Read the model definition and answer for the solid it produces. Units are mm, in the model's axes. A direction names the side the tool comes from. Coordinates: 2 decimals unless noted, no trailing zeros. Write each loop counter-clockwise with the first axis right and the second up, starting at its lowest first coordinate (ties: lowest second). Pieces come first, ordered by that corner, then holes. Notation, with made-up numbers: (-28.5, 50.5) -> (27.5, 50.5) arc R29 ccw to (27.5, 81.5) -> close; hole circle Ø11 at (-25, -36.75). An arc over 180 degrees is marked (long way). Use CSV: the item, a comma, the result in double quotes. Start each with the question number.
from build123d import *

# Parameters (mm, degrees)
BOSS_EXTRUDE1_DEPTH        = 2.5
SKETCH6_W                  = 0.64
SKETCH6_H                  = 0.64
CUT_EXTRUDE1_DEPTH         = 2.5
SKETCH15_W                 = 0.64
SKETCH15_H                 = 0.64
CHAMFER4_SIZE              = 0.12
LPATTERN5_COUNT            = 2
LPATTERN5_PITCH            = 2.5
CHAMFER4_OF_LPATTERN5_SIZE = 0.12


with BuildPart() as part:
    # Sketch4 → Boss-Extrude1 (new body)
    with BuildSketch(Plane(origin=(0, 0, 0), x_dir=(1, 0, 0), z_dir=(0, 1, 0))):
        Polygon((-2.37, -0.9), (-2.37, -0.95), (-2.07, -1.25), (-0.47, -1.25), (-0.17, -0.95), (-0.17, -0.9), (0, -0.9), (0, 0.9), (-0.17, 0.9), (-0.17, 0.95), (-0.47, 1.25), (-2.07, 1.25), (-2.37, 0.95), (-2.37, 0.9), (-2.54, 0.9), (-2.54, -0.9), align=None)
    boss_extrude1 = extrude(amount=BOSS_EXTRUDE1_DEPTH)

    # Sketch6 → Cut-Extrude1 (cut)
    with BuildSketch(Plane.XZ):
        with Locations((-1.27, 0)):
            Rectangle(SKETCH6_W, SKETCH6_H)
        with Locations((1.27, 0)):
            Rectangle(SKETCH6_W, SKETCH6_H)
    extrude(amount=-CUT_EXTRUDE1_DEPTH, mode=Mode.SUBTRACT)

    # Sweep1: sweep along a path in Sketch17
    with BuildLine(Plane(origin=(0, 0, 0), x_dir=(1, 0, 0), z_dir=(0, 0, -1))) as sweep1_path:
        Line((-1.27, 6), (-1.27, -4))
        ThreePointArc((-1.27, -4), (-1.416446609, -4.353553391), (-1.77, -4.5))
        Line((-1.77, -4.5), (-5.52, -4.5))
    # Sketch15 → Sweep1 (sweep)
    with BuildSketch(Plane(origin=(0, -6, 0), x_dir=(1, 0, 0), z_dir=(0, 1, 0))):
        with Locations((-1.27, 0)):
            Rectangle(SKETCH15_W, SKETCH15_H)
    sweep1 = sweep(path=sweep1_path.line)

    # Chamfer4
    chamfer4_edges = [part.edges().sort_by_distance(p)[0] for p in [
        (-0.95, -6, 0),
        (-1.59, -6, 0),
        (-1.27, -6, -0.32),
        (-1.27, -6, 0.32),
        (-5.52, 4.18, 0),
        (-5.52, 4.5, 0.32),
        (-5.52, 4.82, 0),
        (-5.52, 4.5, -0.32),
    ]]
    chamfer(chamfer4_edges, length=CHAMFER4_SIZE)

    # LPattern5: Boss-Extrude1, Sweep1 ×2
    with Locations(*[(0, 0, i * LPATTERN5_PITCH) for i in range(1, LPATTERN5_COUNT)]):
        add(boss_extrude1)
        add(sweep1)

    # Chamfer4 of LPattern5
    chamfer4_of_lpattern5_edges = [part.edges().sort_by_distance(p)[0] for p in [
        (-0.95, -6, 2.5),
        (-1.59, -6, 2.5),
        (-1.27, -6, 2.18),
        (-1.27, -6, 2.82),
        (-5.52, 4.18, 2.5),
        (-5.52, 4.5, 2.82),
        (-5.52, 4.82, 2.5),
        (-5.52, 4.5, 2.18),
    ]]
    chamfer(chamfer4_of_lpattern5_edges, length=CHAMFER4_OF_LPATTERN5_SIZE)


solid = part.part
1) Section A-A, the plane x = -4.05 is taken. Give the vertices of the cut face in (y, z), plus the area to 3 significant figures.
2) The mould has two halves that part along Z. Classify faces 1 (the face through (0, 1, 3)), 2 (the face through (-2.6, 4.4, -0.32)), 3 (the face through (-2.7, 4.4, 0.32)), 4 (the face through (-1, 1, 3.75)): pulls with the +Z half, pulls with the -Z half, needs draft (parallel to the pull), parting line crosses it, or undercut.
3) Find the intervals of material crossed by line 1 along Y through (x, z) = (-2.3, 2.5); line 2 along Y through (x, z) = (-2.65, 2.65); line 3 along Y through (x, z) = (-0.6, 0), in increasing order.
4) Which of the six approach directions +Z, -Z, +X, -X, +Y, -Y give full straight-line access (tool end or side, diameter ignored) to faces 5 (the face through (-2.6, 4.4, 2.18)), 6 (the face through (-2.54, 1, 0)), 7 (the face through (-1.18, 4.57, 0)), 8 (the face through (-2.7, 4.4, 2.82))?
5) Section C-C, the plane y = -3.75 is taken. Give the vertices of the cut face in (x, z), plus the area to 3 significant figures.
6) Section D-D, the plane z = 0.05 is taken. Give the vertices of the cut face in (x, y), plus the area to 3 significant figures.
7) Each of these flat-tipped pins is pushed along its axis until it touches: pin 1 (2.5 mm diameter, centred on x = -4, y = 4, fed in from +Z); pin 2 (1 mm diameter, centred on x = -3.5, z = 2, fed in from -Y); pin 3 (2.5 mm diameter, centred on x = -3.5, y = 4, fed in from -Z). Where does it stop, or does it pass through?
8) Section B-B, the plane x = -1.9 is taken. Give the vertices of the cut face in (y, z), plus the area to 3 significant figures.
The answers:
1,outline,"(4.18, -0.32) -> (4.82, -0.32) -> (4.82, 0.32) -> (4.18, 0.32) -> close; (4.18, 2.18) -> (4.82, 2.18) -> (4.82, 2.82) -> (4.18, 2.82) -> close"
1,area,"0.819 mm^2"
2,face 1,"needs draft"
2,face 2,"pulls with the -Z half"
2,face 3,"undercut"
2,face 4,"pulls with the +Z half"
3,line 1,"y = 0 to 2.5, 4.18 to 4.82"
3,line 2,"y = 4.18 to 4.82"
3,line 3,"y = 0 to 2.5"
4,face 5,"+X, -X, +Y"
4,face 6,"+Z, -Z, -X, -Y"
4,face 7,"+Z, -Z, +X, +Y"
4,face 8,"+Z, +X, -X, +Y"
5,outline,"(-1.59, -0.32) -> (-0.95, -0.32) -> (-0.95, 0.32) -> (-1.59, 0.32) -> close; (-1.59, 2.18) -> (-0.95, 2.18) -> (-0.95, 2.82) -> (-1.59, 2.82) -> close"
5,area,"0.819 mm^2"
6,outline,"(-5.52, 4.3) -> (-5.4, 4.18) -> (-1.77, 4.18) arc R0.18 cw to (-1.59, 4) -> (-1.59, 2.5) -> (-2.54, 2.5) -> (-2.54, 0) -> (-1.59, 0) -> (-1.59, -5.88) -> (-1.47, -6) -> (-1.07, -6) -> (-0.95, -5.88) -> (-0.95, 0) -> (0, 0) -> (0, 2.5) -> (-0.95, 2.5) -> (-0.95, 4) arc R0.82 ccw to (-1.77, 4.82) -> (-5.4, 4.82) -> (-5.52, 4.7) -> close"
6,area,"14.0 mm^2"
7,pin 1,"stops at z = 2.82"
7,pin 2,"stops at y = 4.18"
7,pin 3,"stops at z = -0.32"
8,outline,"(0, -1.25) -> (2.5, -1.25) -> (2.5, 3.75) -> (0, 3.75) -> close; (4.18, -0.32) -> (4.82, -0.32) -> (4.82, 0.32) -> (4.18, 0.32) -> close; (4.18, 2.18) -> (4.82, 2.18) -> (4.82, 2.82) -> (4.18, 2.82) -> close"
8,area,"13.3 mm^2"
